Geometry check sheet. Reference: the model listing, model coordinates, mm. A direction names the side the tool comes from. Coordinates: 2 decimals unless noted, no trailing zeros. Loops run counter-clockwise (first coordinate to the right, second up) from the corner with the lowest first, then second, coordinate; pieces in that order, holes last.
Autodesk Inventor part; units mm, degrees
ref_plane "to_bearing_XY" through (0, 30, -4) normal (0, 0, 1) x (1, 0, 0)
ref_plane "to_bearing_YZ" through (0, 30, -4) normal (1, 0, 0) x (0, 1, 0)
ref_plane "to_bearing_ZX" through (0, 30, -4) normal (0, 1, 0) x (0, 0, 1)
sketch "Sketch_1" plane through (0, 0, 0) normal (0, 0, 1) x (1, 0, 0)
  line L0 (-34, 14) -> (-34, 0)
  line L1 (-34, 0) -> (34, 0)
  line L2 (34, 0) -> (34, 14)
  arc A0 (34, 14) -> (33, 15) centre (33, 14) ccw
  line L3 (33, 15) -> (21, 15)
  arc A1 (20, 16) -> (21, 15) centre (21, 16) ccw
  line L4 (20, 16) -> (20, 34)
  arc A2 (20, 34) -> (4, 50) centre (4, 34) ccw
  line L5 (4, 50) -> (-4, 50)
  arc A3 (-4, 50) -> (-20, 34) centre (-4, 34) ccw
  line L6 (-20, 34) -> (-20, 16)
  arc A4 (-21, 15) -> (-20, 16) centre (-21, 16) ccw
  line L7 (-21, 15) -> (-33, 15)
  arc A5 (-33, 15) -> (-34, 14) centre (-33, 14) ccw
extrude "Extrusion1" add sketch "Sketch_1" along normal mid plane 12
sketch "Sketch_2" plane through (0, 0, 0) normal (1, 0, 0) x (0, 0, -1)
  line L0 (6, 30) -> (-6, 30)
  line L1 (-6, 30) -> (-6, 44)
  line L2 (-6, 44) -> (-4.35, 44)
  line L3 (-4.35, 44) -> (-4.35, 44.7)
  line L4 (-4.35, 44.7) -> (-3, 44.7)
  line L5 (-3, 44.7) -> (-3, 44)
  line L6 (-3, 44) -> (4, 44)
  line L7 (4, 44) -> (4, 42.5)
  line L8 (4, 42.5) -> (6, 42.5)
  line L9 (6, 42.5) -> (6, 30)
  line L10 (6, 30) -> (-6, 30)
revolve "Revolution1" cut sketch "Sketch_2" angle 360 about axis through (0, 30, -6) along (0, 0, -1)
sketch "Sketch3" plane through (-34, 0, 6) normal (0, -1, 0) x (1, 0, 0)
  point P0 (61, -6)
hole "Hole1" at (27, 0, 0) direction (0, 1, 0) diameter 6.5 depth 15
pattern_linear "Rectangular Pattern1" count 2 spacing 54 along (-1, 0, 0) of "Hole1"
ref_plane "to_bearing_XY" through (0, 30, -4) normal (0, 0, 1) x (1, 0, 0)
ref_plane "to_bearing_YZ" through (0, 30, -4) normal (1, 0, 0) x (0, 1, 0)
ref_plane "to_bearing_ZX" through (0, 30, -4) normal (0, 1, 0) x (0, 0, 1)
ref_plane "to_snapring_XY" through (0, 30, 4.35) normal (0, 0, 1) x (1, 0, 0)
ref_plane "to_snapring_YZ" through (0, 30, 4.35) normal (1, 0, 0) x (0, 1, 0)
ref_plane "to_snapring_ZX" through (0, 30, 4.35) normal (0, 1, 0) x (0, 0, 1)
properties part number "C-BGHKA6902ZZ-30_b_b"
(1) Sectioned sample at D-D on y = 6. Record the cut outline in (x, z).
Findings:
outline: (-34, -6) - (34, -6) - (34, 6) - (-34, 6) - close; hole circle Ø6.5 at (-27, 0); hole circle Ø6.5 at (27, 0)
(2) Sectioned sample at C-C on y = 30. Record the cut outline in (x, z).
Findings:
outline: (-20, -6) - (-12.5, -6) - (-12.5, -4) - (-14, -4) - (-14, 3) - (-14.7, 3) - (-14.7, 4.35) - (-14, 4.35) - (-14, 6) - (-20, 6) - close; (12.5, -6) - (20, -6) - (20, 6) - (14, 6) - (14, 4.35) - (14.7, 4.35) - (14.7, 3) - (14, 3) - (14, -4) - (12.5, -4) - close
(3) Sectioned sample at A-A on z = 0. Record the cut outline in (x, y).
Findings:
outline: (-34, 0) - (-30.25, 0) - (-30.25, 15) - (-33, 15) arc R1 ccw to (-34, 14) - close; (-23.75, 0) - (23.75, 0) - (23.75, 15) - (21, 15) arc R1 cw to (20, 16) - (20, 34) arc R16 ccw to (4, 50) - (-4, 50) arc R16 ccw to (-20, 34) - (-20, 16) arc R1 cw to (-21, 15) - (-23.75, 15) - close; (30.25, 0) - (34, 0) - (34, 14) arc R1 ccw to (33, 15) - (30.25, 15) - close; hole circle Ø28 at (0, 30)
(4) Draft check along X on faces 1 (the flat face through (-30, 15, -3)), 2 (the cylindrical face through (30.173, 7.605, 0.705)), 3 (the cylindrical face through (15.189, 45.437, -0.084)). Enter one of: +X half, -X half, draft (parallel to the pull), parting line (faces both ways), or undercut.
Findings:
face 1: draft
face 2: undercut
face 3: +X half
(5) Scan lines: L1, parallel to X at y = 14, z = -0.25; L2, parallel to X at y = 10, z = -1; L3, parallel to Z at x = 27, y = 7. Record each from-to range of solid material in increasing order.
Findings:
L1: x = -34 to -30.24, -23.76 to 23.76, 30.24 to 34
L2: x = -34 to -30.09, -23.91 to 23.91, 30.09 to 34
L3: z = -6 to -3.25, 3.25 to 6
(6) Access from +Z, -Z, +X, -X, +Y, -Y to the whole of each face (thin tool, end or side, straight path). Record for faces 4 (the flat face through (20, 25, 0)), 5 (the flat face through (-12, 38, 4.35)), 6 (the flat face through (11.5, 24.7, -4)).
Findings:
face 4: +Z, -Z, +X, +Y
face 5: none
face 6: +Z
(7) Gauge pin test, flat ends, axial feed: pin 1 Ø4 at (y, z) = (17.5, 3.5) entering from +X; pin 2 Ø3.5 at (x, z) = (-26.5, 2.5) entering from +Y; pin 3 Ø1.5 at (y, z) = (23.5, 2.5) entering from -X. Record the tip position at first contact, or that the pin passes through.
Findings:
pin 1: stops at x = 20.13
pin 2: stops at y = 15
pin 3: stops at x = -20
(8) Sectioned sample at B-B on x = 0. Record the cut outline in (y, z).
Findings:
outline: (0, -6) - (17.5, -6) - (17.5, -4) - (16, -4) - (16, 3) - (15.3, 3) - (15.3, 4.35) - (16, 4.35) - (16, 6) - (0, 6) - close; (42.5, -6) - (50, -6) - (50, 6) - (44, 6) - (44, 4.35) - (44.7, 4.35) - (44.7, 3) - (44, 3) - (44, -4) - (42.5, -4) - close
